The figure shows three views and two pictorial views of one solid part (mm, origin at its lowest corner). Answer the questions. Coordinates: 2 decimals unless noted, no trailing zeros. Order: outer loops, then holes, each group sorted by start corner. A loop starts at its lowest first (then second) coordinate and runs counter-clockwise, first axis right, second up. Notation, with made-up numbers: (-26.5, 88.5) -> (-12.5, 88.5) arc R27 ccw to (-12.5, 111.5) -> close; hole circle Ø7 at (-7, -11). An arc over 180 degrees is marked (long way). Write item = value, one per line. Start each with the question number.
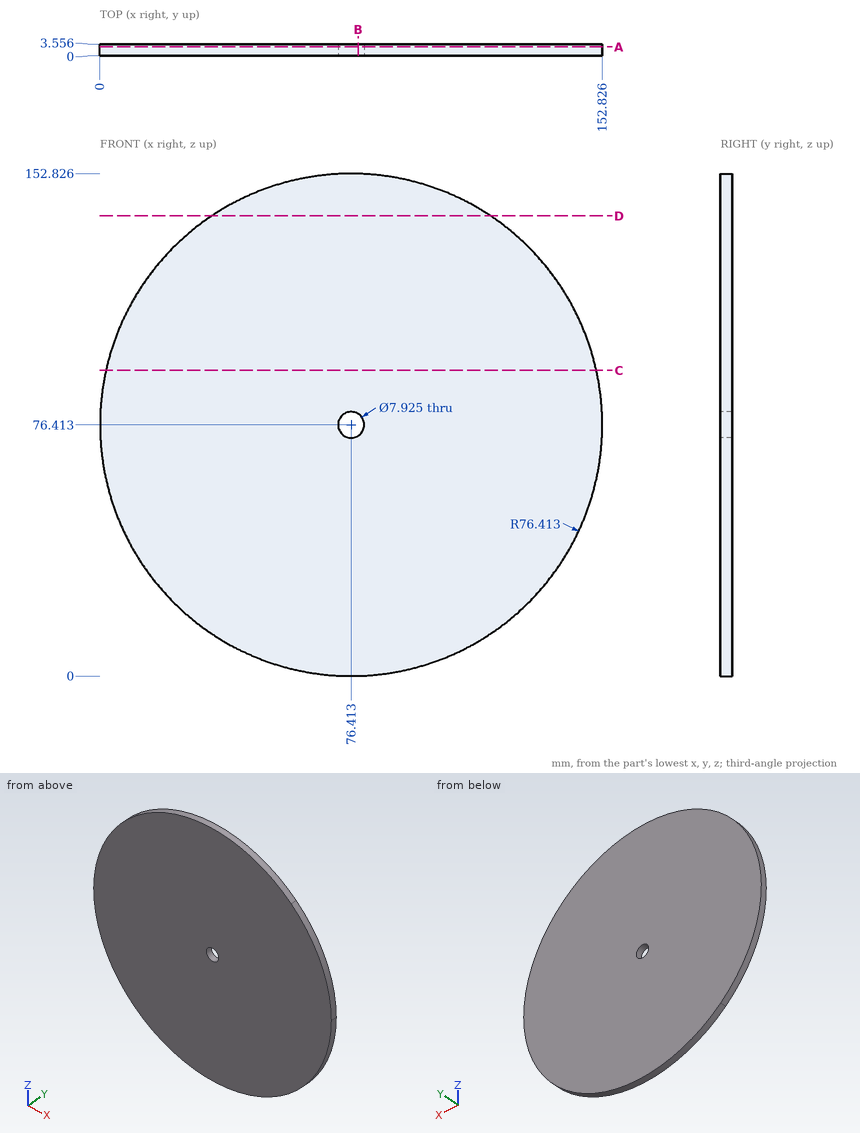
Item 1: Section B-B, the plane x = 78.5 is taken. Give the vertices of the cut face in (y, z) (1 decimal).
Item 2: Each of these flat-tipped pins is pushed along its axis until it touches: pin 1 (5 mm diameter, centred on x = 76.41, z = 76.41, fed in from +Y); pin 2 (1 mm diameter, centred on y = 2.5, z = 104.5, fed in from +X); pin 3 (2 mm diameter, centred on y = 1.5, z = 74.5, fed in from -X); pin 4 (2 mm diameter, centred on y = 2, z = 96.5, fed in from +X). Where does it stop, or does it pass through?
Item 3: Section D-D, the plane z = 140 is taken. Give the vertices of the cut face in (x, y).
Item 4: Consider probe 1 along Z at (x, y) = (75, 0.2) (1 decimal); probe 2 along X at (y, z) = (3.4, 80) (1 decimal); probe 3 along X at (y, z) = (2.05, 75.5) (1 decimal). Determine where each line is inside the solid, lowest interval first.
Item 5: Section A-A, the plane y = 2.7 is taken. Give the vertices of the cut face in (x, z) (1 decimal).
Item 6: Section C-C, the plane z = 93 is taken. Give the vertices of the cut face in (x, y).
A:
q1.outline = (0, 0) -> (3.6, 0) -> (3.6, 73) -> (0, 73) -> close; (0, 79.8) -> (3.6, 79.8) -> (3.6, 152.8) -> (0, 152.8) -> close
q2.pin_1 = through
q2.pin_2 = 147.67
q2.pin_3 = 0.01
q2.pin_4 = 150.4
q3.outline = (34.04, 0) -> (118.79, 0) -> (118.79, 3.56) -> (34.04, 3.56) -> close
q4.probe_1 = 0 to 72.7, 80.1 to 152.8
q4.probe_2 = 0.1 to 74.7, 78.1 to 152.7
q4.probe_3 = 0 to 72.6, 80.3 to 152.8
q5.outline = (26.1, 18.9) arc R76.4 ccw to (125.5, 17.8) arc R76.4 ccw to (152.8, 76.4) arc R76.4 ccw to (127, 133.7) arc R76.4 ccw to (27.4, 135) arc R76.4 ccw to start; hole circle Ø7.9 at (76.4, 76.4)
q6.outline = (1.82, 0) -> (151, 0) -> (151, 3.56) -> (1.82, 3.56) -> close
